from build123d import *

# Parameters (mm, degrees)
SKETCH_1_R      = 35
SKETCH_1_R_2    = 5
EXTRUDE_1_DEPTH = 3


with BuildPart() as part:
    # 스케치1 → 보스-돌출1 (new body)
    with BuildSketch(Plane.XY):
        Circle(SKETCH_1_R)
        with BuildLine():
            ThreePointArc((32.5, 0), (30, -2.5), (27.5, 0))
            ThreePointArc((27.5, 0), (19.445436483, 19.445436483), (0, 27.5))
            ThreePointArc((0, 27.5), (-2.5, 30), (0, 32.5))
            ThreePointArc((0, 32.5), (22.980970389, 22.980970389), (32.5, 0))
        make_face(mode=Mode.SUBTRACT)
        with BuildLine():
            ThreePointArc((0, -27.5), (2.5, -30), (0, -32.5))
            ThreePointArc((0, -32.5), (-22.980970405, -22.980970372), (-32.5, 4.6e-08))
            ThreePointArc((-32.5, 4.6e-08), (-29.999999977, 2.5), (-27.5, 0))
            ThreePointArc((-27.5, 0), (-19.445436483, -19.445436483), (0, -27.5))
        make_face(mode=Mode.SUBTRACT)
        Circle(SKETCH_1_R_2, mode=Mode.SUBTRACT)
    extrude(amount=EXTRUDE_1_DEPTH)


solid = part.part
Input: part model. Units: mm. Frame: model coordinates. A direction names the side the tool comes from. Round coordinates to 2 decimals unless told otherwise and drop trailing zeros. Order: outer loops, then holes, each group sorted by start corner. A loop starts at its lowest first (then second) coordinate and runs counter-clockwise, first axis right, second up. Notation, with made-up numbers: (38.5, -29) - (65.5, -29) arc R15 ccw to (65.5, 0) - close; hole circle Ø11 at (43.5, -36). An arc over 180 degrees is marked (long way). Answer as a JSON object with one key per item and string values. Group by question number.
(1) Cut plane B-B (x = 14.5). Return loops of the section in (y, z).
(2) Cut plane A-A (z = 0.7). Return loops of the section in (x, y).
(3) Cut plane D-D (y = -1). Return loops of the section in (x, z).
(4) Draft query along Y for faces 3 (the face through (0, -7, 3)), 4 (the face through (-28, -21, 1)), 5 (the face through (19.66, 19.23, 1.48)). Return one class per face: released by +Y, released by -Y, zero draft, split by the parting line, or undercut.
(5) Material intervals for probe 1 along Y at (x, z) = (-1, 0.3); probe 2 along Y at (x, z) = (-16, 0.95); probe 3 along Y at (x, z) = (-21.5, 0.25), sorted ascending. Write a range as from..to.
(6) Reachability of faces 1 (the face through (0, -7, 0)), 2 (the face through (-30.1, 2.5, 1.5)) from +Z, -Z, +X, -X, +Y, -Y: full face, straight path, thin tool, end or side. Return the list, or none.
(7) Cut plane C-C (y = -10). Return loops of the section in (x, z), then the cut area to 3 significant figures.
Here are the results:
{
 "1": {"outline": "(-31.86, 0) - (23.37, 0) - (23.37, 3) - (-31.86, 3) - close; (29.09, 0) - (31.86, 0) - (31.86, 3) - (29.09, 3) - close"},
 "2": {"outline": "circle Ø70 at (0, 0); hole (-32.5, 0) arc R32.5 ccw to (0, -32.5) arc R2.5 ccw to (0, -27.5) arc R27.5 cw to (-27.5, 0) arc R2.5 ccw to start; hole circle Ø10 at (0, 0); hole (0, 27.5) arc R27.5 cw to (27.5, 0) arc R2.5 ccw to (32.5, 0) arc R32.5 ccw to (0, 32.5) arc R2.5 ccw to start"},
 "3": {"outline": "(-34.99, 0) - (-32.48, 0) - (-32.48, 3) - (-34.99, 3) - close; (-27.48, 0) - (-4.9, 0) - (-4.9, 3) - (-27.48, 3) - close; (4.9, 0) - (27.71, 0) - (27.71, 3) - (4.9, 3) - close; (32.29, 0) - (34.99, 0) - (34.99, 3) - (32.29, 3) - close"},
 "4": {"face 3": "zero draft", "face 4": "split by the parting line", "face 5": "undercut"},
 "5": {"probe 1": "y = -34.99..-32.48, -27.48..-4.9, 4.9..27.71, 32.29..34.99", "probe 2": "y = -31.13..-28.29, -22.37..31.13", "probe 3": "y = -27.62..-24.37, -17.15..27.62"},
 "6": {"face 1": "-Z, +X, -X, +Y, -Y", "face 2": "+Z, -Z"},
 "7": {"outline": "(-33.54, 0) - (-30.92, 0) - (-30.92, 3) - (-33.54, 3) - close; (-25.62, 0) - (33.54, 0) - (33.54, 3) - (-25.62, 3) - close", "area": "185 mm^2"}
}
